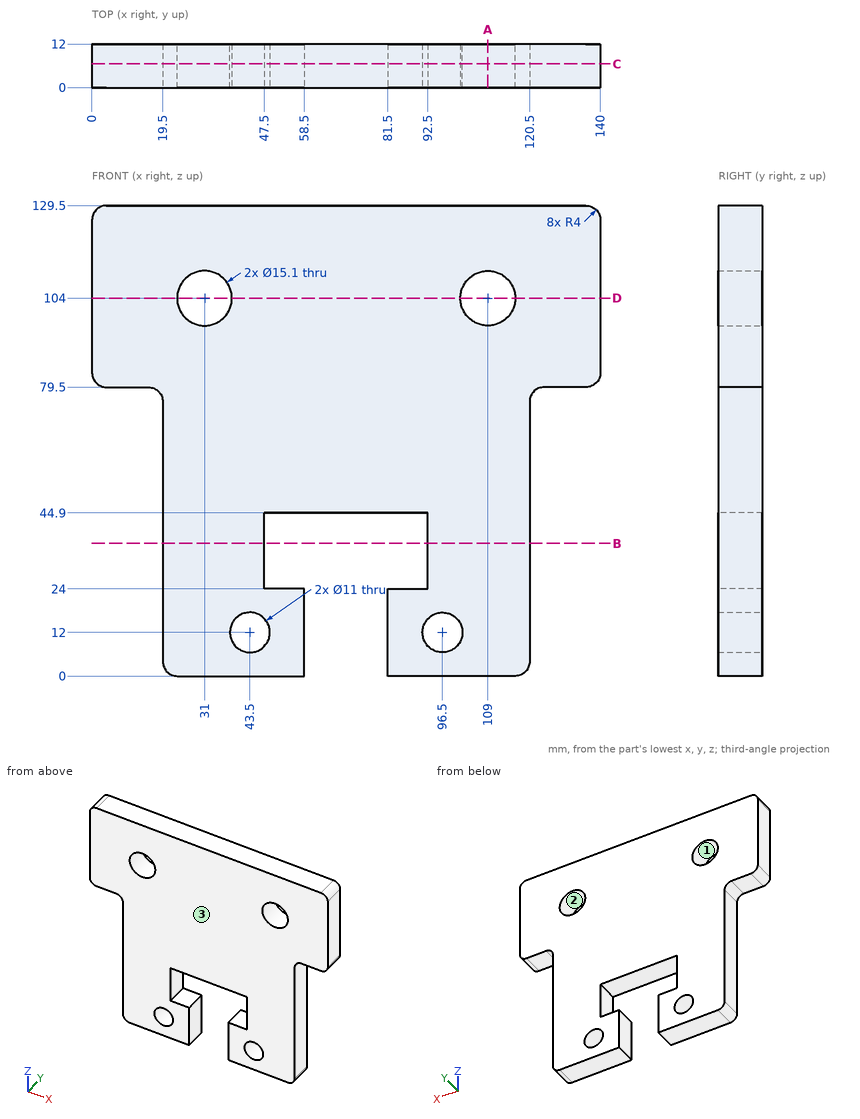
Print and shaded views of the part. All mm, measured from the part's lowest x, y and z. Give positions to 0.01 mm unless a question says otherwise; leave off trailing zeros. Write each loop counter-clockwise with the first axis right and the second up, starting at its lowest first coordinate (ties: lowest second). Pieces come first, ordered by that corner, then holes. Notation, with made-up numbers: (-6.5, 0.25) -> (-0.5, 0.25) arc R18 ccw to (-0.5, 31.25) -> close; hole circle Ø7 at (25.25, 78). An arc over 180 degrees is marked (long way). Use CSV: the item, a comma, the result in double quotes. Start each with the question number.
1) Cut at B-B on z = 36.5. List the corners of the cut face in (x, y).
2) Cut at D-D on z = 104. List the corners of the cut face in (x, y).
3) Cut at A-A on x = 109. List the corners of the cut face in (y, z).
4) Drill centre lines: L1, parallel to Z at x = 109, y = 4; L2, parallel to X at y = 11, z = 22.5; L3, parallel to X at y = 3, z = 108.5. Where is each one in solid material? Low to high.
5) Pin check, flat tips, straight feed: P1, Ø6, axis at x = 7.5, y = 7.5, coming from the -Z side; P2, Ø4, axis at y = 9, z = 33.5, coming from the +X side; P3, Ø6, axis at y = 6.5, z = 35.5, coming from the -X side. Stop position of each tip, or through.
6) Cut at C-C on y = 6.5. List the corners of the cut face in (x, z), plus the area to 3 significant figures.
7) Two-plate mould, pull along X, no slides. Class the marked faces 1, 2 and 3: released by +X, released by -X, zero draft, split by the parting line, or undercut.
Final values:
1,outline,"(19.5, 0) -> (47.5, 0) -> (47.5, 12) -> (19.5, 12) -> close; (92.5, 0) -> (120.5, 0) -> (120.5, 12) -> (92.5, 12) -> close"
2,outline,"(0, 0) -> (23.45, 0) -> (23.45, 12) -> (0, 12) -> close; (38.55, 0) -> (101.45, 0) -> (101.45, 12) -> (38.55, 12) -> close; (116.55, 0) -> (140, 0) -> (140, 12) -> (116.55, 12) -> close"
3,outline,"(0, 0) -> (12, 0) -> (12, 96.45) -> (0, 96.45) -> close; (0, 111.55) -> (12, 111.55) -> (12, 129.5) -> (0, 129.5) -> close"
4,L1,"z = 0 to 96.45, 111.55 to 129.5"
4,L2,"x = 19.5 to 58.5, 81.5 to 120.5"
4,L3,"x = 0 to 24.94, 37.06 to 102.94, 115.06 to 140"
5,P1,"stops at z = 79.5"
5,P2,"stops at x = 120.5"
5,P3,"stops at x = 19.5"
6,outline,"(0, 83.5) arc R4 ccw to (4, 79.5) -> (15.5, 79.5) arc R4 cw to (19.5, 75.5) -> (19.5, 4) arc R4 ccw to (23.5, 0) -> (58.5, 0) -> (58.5, 24) -> (47.5, 24) -> (47.5, 44.9) -> (92.5, 44.9) -> (92.5, 24) -> (81.5, 24) -> (81.5, 0) -> (116.5, 0) arc R4 ccw to (120.5, 4) -> (120.5, 75.5) arc R4 cw to (124.5, 79.5) -> (136, 79.5) arc R4 ccw to (140, 83.5) -> (140, 125.5) arc R4 ccw to (136, 129.5) -> (4, 129.5) arc R4 ccw to (0, 125.5) -> close; hole circle Ø15.1 at (31, 104); hole circle Ø11 at (43.5, 12); hole circle Ø11 at (96.5, 12); hole circle Ø15.1 at (109, 104)"
6,area,"13,000 mm2"
7,face 1,"undercut"
7,face 2,"undercut"
7,face 3,"zero draft"
